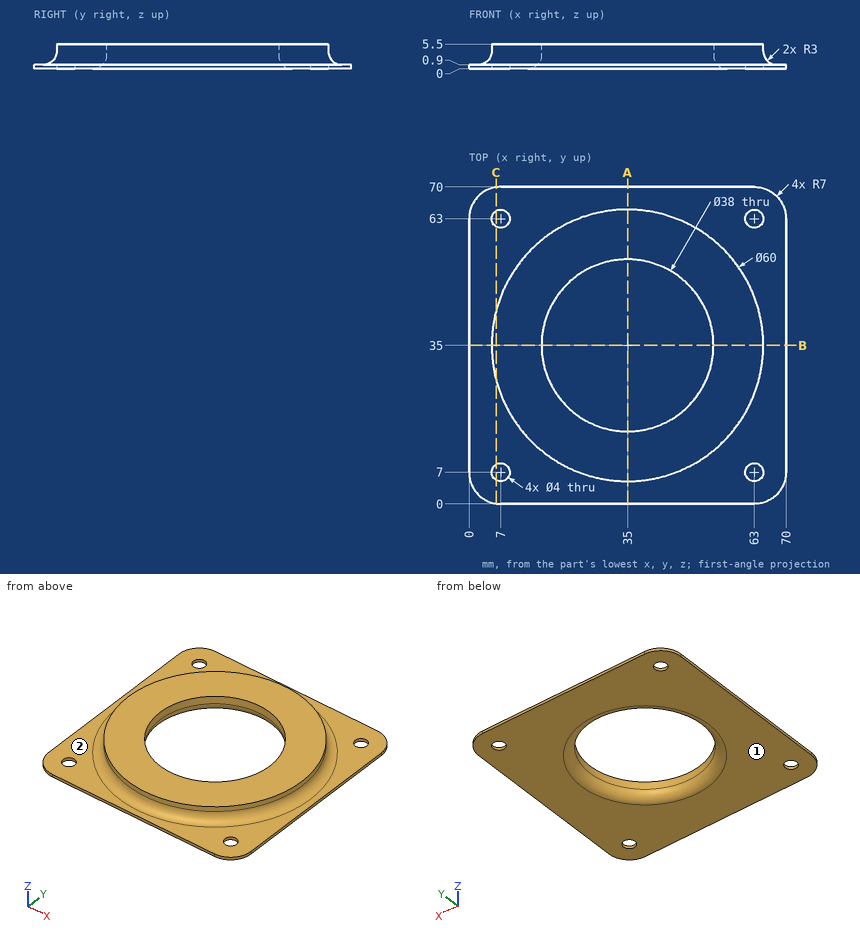
Could you check a few things on this drawing? It's one solid part, dimensions in mm from its lowest x, y, z. A direction names the side the tool comes from. Give positions to 0.01 mm unless a question says otherwise; leave off trailing zeros. Write each loop counter-clockwise with the first axis right and the second up, starting at its lowest first coordinate (ties: lowest second). Pieces come first, ordered by that corner, then holes. Notation, with made-up numbers: M 55,86.5 L 68,86.5 A19 ccw 68,110.5 Z; hole C 38,14 d5. An arc over 180 degrees is marked long. Put each result on its own line as item: value. Start each with the question number.
Item 1: Will these pins go through, and if not, where does the flat tip stop? pin 1 (4.5 mm diameter, centred on x = 63, y = 63, fed in from +Z); pin 2 (2 mm diameter, centred on y = 46, z = 2.5, fed in from +X).
Item 2: I need wall thicknesses on L1, parallel to Y at x = 63, z = 0.2; L2, parallel to Z at x = 55.5, y = 3.5. Which ranges of each line are inside material? Lowest first, please. Write a range as from..to.
Item 3: If we section it at A-A, the plane x = 35: Write out the boundary of the cut face in (y, z), then the cut area to 3 significant figures.
Item 4: If we section it at C-C, the plane x = 6: Count the separate pieces of the cut face and the enclosed holes in it, then the cut area to 3 significant figures.
Item 5: On a 3-axis mill with a long thin cutter (end or side, diameter ignored), from which of +Z, -Z, +X, -X, +Y, -Y can I reach the whole of each face in a straight line? I mean the marked faces 1 and 2. Say none if no direction works.
Values:
1. pin 1: z = 0.9
1. pin 2: x = 64.25
2. L1: 0..5, 9..61, 65..70
2. L2: 0..0.9
3. outline: M 0,0 L 13,0 A3 ccw 16,3 L 16,5.5 L 5,5.5 L 5,3.9 A3 cw 2,0.9 L 0,0.9 Z; M 54,3 A3 ccw 57,0 L 70,0 L 70,0.9 L 68,0.9 A3 cw 65,3.9 L 65,5.5 L 54,5.5 Z
3. area: 130 mm²
4. separate pieces: 3
4. enclosed holes: 0
4. area: 140 mm²
5. face 1: -Z, +X, -X, +Y, -Y
5. face 2: +Z
